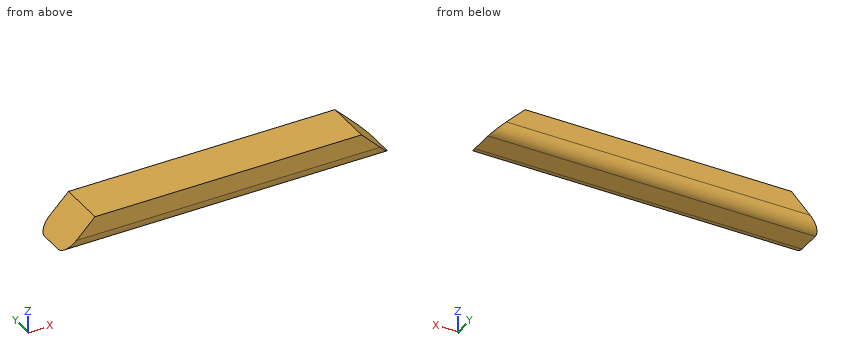
from build123d import *

# Parameters (mm, degrees)
BOSS_EXTRUDE1_DEPTH = 888.6444
SKETCH2_W           = 344.402501539
SKETCH2_H           = 780.457540958
CUT_EXTRUDE1_DEPTH  = 59.371664787


with BuildPart() as part:
    # Sketch1 → Boss-Extrude1 (new body)
    with BuildSketch(Plane(origin=(0, 0, 0), x_dir=(0, 0, -1), z_dir=(1, 0, 0))):
        with BuildLine():
            Line((0, 0), (31.75, 0))
            ThreePointArc((31.75, 0), (54.200640303, 9.299359697), (63.5, 31.75))
            Line((63.5, 31.75), (63.5, 95.25))
            ThreePointArc((63.5, 95.25), (54.200640303, 117.700640303), (31.75, 127))
            Line((31.75, 127), (0, 127))
            Line((0, 127), (-19.05, 127))
            Line((-19.05, 127), (-19.05, 0))
            Line((-19.05, 0), (0, 0))
        make_face()
    extrude(amount=BOSS_EXTRUDE1_DEPTH)

    # Sketch2 → Cut-Extrude1 (cut, through all)
    with BuildSketch(Plane(origin=(412.5722, 0, 412.5722), x_dir=(0, 1, 0), z_dir=(0.707106781, 0, 0.707106781))):
        with Locations((32.995160032, -673.267761909)):
            Rectangle(SKETCH2_W, SKETCH2_H)
    cut_extrude1 = extrude(amount=CUT_EXTRUDE1_DEPTH, mode=Mode.SUBTRACT)

    # Mirror1: Cut-Extrude1 across plane
    add(cut_extrude1.mirror(Plane(origin=(444.3222, 0, 0), x_dir=(0, 0, 1), z_dir=(1, 0, 0))), mode=Mode.SUBTRACT)


solid = part.part
Geometry: final body of the model. Coordinates: model frame, mm. Give positions to 0.01 mm unless a question says otherwise; leave off trailing zeros. Write each loop counter-clockwise with the first axis right and the second up, starting at its lowest first coordinate (ties: lowest second). Pieces come first, ordered by that corner, then holes. Notation, with made-up numbers: (-22, -1) - (-18, -1) arc R27 ccw to (-18, 30) - close; hole circle Ø10 at (84, -5). An arc over 180 degrees is marked (long way). Return JSON: item names as keys, results as strings. Group by question number.
1) Section A-A on x = 454.5. Return the cut outline in (y, z).
2) Section B-B on y = 55.5. Return the cut outline in (x, z).
3) Section C-C on z = -47. Return the cut outline in (x, y), plus the area to 3 significant figures.
4) First-contact query: P1, Ø8, axis at y = 32, z = -13, coming from the -X side; P2, Ø2, axis at x = 182.5, z = -10, coming from the -Y side; P3, Ø4, axis at y = 93.5, z = 7.5, coming from the +X side; P4, Ø10, axis at y = 77, z = -48, coming from the -X side. Flat tips, straight axial feed; report the tip coordinate or a pass-through.
5) Line query: line 1 (X direction, y = 86.5, z = 11); line 2 (X direction, y = 85.5, z = -6); line 3 (Y direction, x = 538, z = -47). Output: solid intervals per line, ascending.
Filled in:
{
 "1": {"outline": "(0, -31.75) arc R31.75 ccw to (31.75, -63.5) - (95.25, -63.5) arc R31.75 ccw to (127, -31.75) - (127, 19.05) - (0, 19.05) - close"},
 "2": {"outline": "(0, -63.5) - (888.64, -63.5) - (806.09, 19.05) - (82.55, 19.05) - close"},
 "3": {"outline": "(16.5, 3.9) - (872.14, 3.9) - (872.14, 123.1) - (16.5, 123.1) - close", "area": "102,000 mm^2"},
 "4": {"P1": "stops at x = 46.5", "P2": "stops at y = 0", "P3": "stops at x = 819.64", "P4": "stops at x = 10.5"},
 "5": {"line 1": "x = 74.5 to 814.14", "line 2": "x = 57.5 to 831.14", "line 3": "y = 3.9 to 123.1"}
}
